from build123d import *

# Parameters (mm, degrees)
SKETCH_1_W          = 32
SKETCH_1_H          = 30
EXTRUDE_1_DEPTH     = 8
SKETCH_2_R          = 6
EXTRUDE_2_DEPTH     = 10
CUT_EXTRUDE_START   = 10
SKETCH_4_R          = 11
CUT_EXTRUDE_1_DEPTH = 7
SKETCH_5_R          = 2.5
CUT_EXTRUDE_2_DEPTH = 44.119202509
CHAMFER_1_SIZE      = 3


with BuildPart() as part:
    # 草图1 → 凸台-拉伸1 (new body)
    with BuildSketch(Plane(origin=(0, 0, 0), x_dir=(1, 0, 0), z_dir=(0, 1, 0))):
        Rectangle(SKETCH_1_W, SKETCH_1_H)
    extrude(amount=EXTRUDE_1_DEPTH)

    # 草图2 → 凸台-拉伸2 (add)
    with BuildSketch(Plane.ZY.offset(16)):
        with BuildLine():
            Line((15, 0), (-15, 0))
            Line((-15, 0), (-15, 30.125))
            ThreePointArc((-15, 30.125), (0, 45.125), (15, 30.125))
            Line((15, 30.125), (15, 0))
        make_face()
        with Locations((0, 30.125)):
            Circle(SKETCH_2_R, mode=Mode.SUBTRACT)
    extrude_2 = extrude(amount=-EXTRUDE_2_DEPTH)

    # 草图4 → 切除-拉伸1 (cut)
    with BuildSketch(Plane.ZY.offset(6).offset(CUT_EXTRUDE_START)):
        with Locations(Location((0, 30.125, 0), (0, 0, 180))):
            Circle(SKETCH_4_R)
    extrude(amount=-CUT_EXTRUDE_1_DEPTH, mode=Mode.SUBTRACT)

    # 镜向1: 凸台-拉伸2 across plane
    add(extrude_2.mirror(Plane(origin=(0, 0, 0), x_dir=(0, 0, 1), z_dir=(1, 0, 0))))

    # 草图5 → 切除-拉伸2 (cut, through all)
    with BuildSketch(Plane(origin=(0, 8, 0), x_dir=(1, 0, 0), z_dir=(0, 1, 0))):
        with Locations(Location((0, 8, 0), (0, 0, 270))):
            Circle(SKETCH_5_R)
        with Locations(Location((0, -8, 0), (0, 0, 270))):
            Circle(SKETCH_5_R)
    extrude(amount=-CUT_EXTRUDE_2_DEPTH, mode=Mode.SUBTRACT)

    # 倒角1
    chamfer_1_edges = [part.edges().sort_by_distance(p)[0] for p in [
        (0, 8, -10.5),
        (0, 8, 5.5),
    ]]
    chamfer(chamfer_1_edges, length=CHAMFER_1_SIZE)


solid = part.part
The listing builds one solid part. Answer for the finished solid, in the listing's coordinates (mm). A direction names the side the tool comes from. Round coordinates to 2 decimals unless told otherwise and drop trailing zeros. Write each loop counter-clockwise with the first axis right and the second up, starting at its lowest first coordinate (ties: lowest second). Pieces come first, ordered by that corner, then holes. Notation, with made-up numbers: M 86.5,0 L 141.5,0 A27 ccw 141.5,28 Z; hole C 11,-17 d7. An arc over 180 degrees is marked long. Write each question's results on one line, items separated by ' | '. Start each with the question number.
(1) Determine the mould class of faces 1 (the flat face through (-16, 17, 0)), 2 (the flat face through (6, 23, 0)), 3 (the cylindrical face through (-11.07, 45.12, -0.33)) for opening direction X: +X half, -X half, draft (parallel to the pull), parting line (faces both ways), or undercut.
(2) The part is cut by section D-D, the plane y = 38. Write down the section's boundary in (x, z).
(3) For faces 4 (the flat face through (0, 8, 0)), 5 (the cylindrical face through (-12.549, 40.863, 2.385)), 6 (the cylindrical face through (11.07, 24.268, -1.301)), determine the directions among +Z, -Z, +X, -X, +Y, -Y from which every point of the face is accessible in a straight line to the end or side of a thin tool.
(4) Find the intervals of material crossed by line 1 (X direction, y = 3.7, z = -8); line 2 (Y direction, x = -10.75, z = 0) (3 decimals); line 3 (X direction, y = 15, z = 13.75), in increasing order.
(5) The part is cut by section B-B, the plane x = 0. Write down the section's boundary in (y, z), and give its area (3 significant figures).
(6) The part is cut by section C-C, the plane y = 3. Write down the section's boundary in (x, z), and give its area (3 significant figures).
(7) Each of these flat-tipped pins is pushed along its axis until it touches: P1, Ø3, axis at y = 38, z = -2.5, coming from the -X side; P2, Ø1, axis at x = -2, z = -7.5, coming from the +Y side; P3, Ø2, axis at x = -7, y = 35, coming from the -Z side. Where does it stop, or does it pass through?
(8) The part is cut by section A-A, the plane z = 0. Write down the section's boundary in (x, y) (3 decimals).
Worked answers:
1) face 1: -X half | face 2: undercut | face 3: draft
2) outline: M -16,-12.77 L -6,-12.77 L -6,12.77 L -16,12.77 L -16,7.68 L -9,7.68 L -9,-7.68 L -16,-7.68 Z; M 6,-12.77 L 16,-12.77 L 16,12.77 L 6,12.77 Z
3) face 4: +Z, -Z, +Y | face 5: -X | face 6: +X, -X
4) line 1: x = -16 to -2.5, 2.5 to 16 | line 2: y = 0 to 19.125, 41.125 to 45.125 | line 3: x = -16 to -6, 6 to 16
5) outline: M 0,-15 L 8,-15 L 8,-13.5 L 5,-10.5 L 0,-10.5 Z; M 0,-5.5 L 5,-5.5 L 8,-2.5 L 8,2.5 L 5,5.5 L 0,5.5 Z; M 0,10.5 L 5,10.5 L 8,13.5 L 8,15 L 0,15 Z | area: 142 mm²
6) outline: M -16,-15 L 16,-15 L 16,15 L -16,15 Z; hole C 0,-8 d5; hole C 0,8 d5 | area: 921 mm²
7) P1: stops at x = -9 | P2: stops at y = 5.06 | P3: stops at z = -14.49
8) outline: M -16,0 L 16,0 L 16,24.125 L 6,24.125 L 6,8 L -6,8 L -6,24.125 L -9,24.125 L -9,19.125 L -16,19.125 Z; M -16,41.125 L -9,41.125 L -9,36.125 L -6,36.125 L -6,45.125 L -16,45.125 Z; M 6,36.125 L 16,36.125 L 16,45.125 L 6,45.125 Z
